Can you work these out from the drawing? Everything is in mm from the part's minimum corner. Give positions to 0.01 mm unless a question says otherwise; leave off trailing zeros. Write each loop counter-clockwise with the first axis right and the second up, starting at its lowest first coordinate (ties: lowest second). Pieces come first, ordered by that corner, then holes. Notation, with made-up numbers: (2, 66.25) - (59, 66.25) arc R24 ccw to (59, 95.25) - close; hole circle Ø11 at (-37, 67.25). An arc over 180 degrees is marked (long way). Use a Markdown table: item, result. Add a question column.
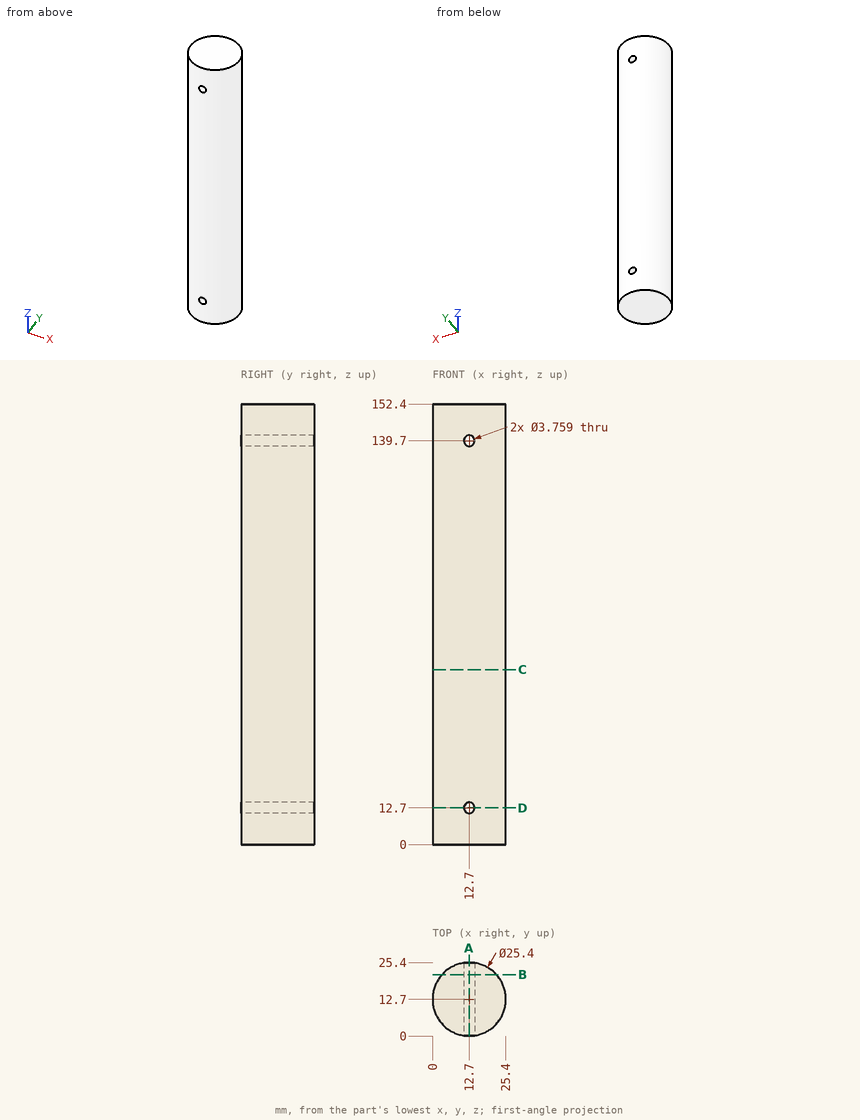
Q1. Suppose I cut it at C-C (z = 60.5). Please give me the cut outline in (x, y).
Q2. If I drill on probe 1 along Z at (x, y) = (12.7, 20); probe 2 along X at (y, z) = (12, 16); probe 3 along X at (y, z) = (17, 130), over which ranges is the centre line in solid material (lowest first)? Write a range as [from, to].
Q3. Suppose I cut it at A-A (x = 12.7). Please give me the cut outline in (y, z).
Q4. I'm going to push flat-ended pins straight in: P1, Ø5, axis at x = 2.5, z = 72.5, coming from the -Y side; P2, Ø2.5, axis at x = 12.7, z = 139.7, coming from the -Y side; P3, Ø6, axis at x = 3.5, z = 50.5, coming from the -Y side; P4, Ø10, axis at y = 5.5, z = 62.5, coming from the -X side. Where does each tip first touch, or does it pass through?
Q5. Suppose I cut it at D-D (z = 12.7). Please give me the cut outline in (x, y).
Q6. Suppose I cut it at B-B (y = 21.25). Please give me the cut outline in (x, z), and give its area (3 significant figures).
Derived:
| question | item | result |
|---|---|---|
| 1 | outline | circle Ø25.4 at (12.7, 12.7) |
| 2 | probe 1 | [0, 10.82], [14.58, 137.82], [141.58, 152.4] |
| 2 | probe 2 | [0.02, 25.38] |
| 2 | probe 3 | [0.75, 24.65] |
| 3 | outline | (0, 0) - (25.4, 0) - (25.4, 10.82) - (0, 10.82) - close; (0, 14.58) - (25.4, 14.58) - (25.4, 137.82) - (0, 137.82) - close; (0, 141.58) - (25.4, 141.58) - (25.4, 152.4) - (0, 152.4) - close |
| 4 | P1 | y = 2.6 |
| 4 | P2 | through |
| 4 | P3 | y = 1.62 |
| 4 | P4 | x = 0.19 |
| 5 | outline | (10.82, 0.14) - (10.82, 25.26) arc R12.7 ccw to start; (14.58, 0.14) arc R12.7 ccw to (14.58, 25.26) - close |
| 6 | outline | (3.31, 0) - (22.09, 0) - (22.09, 152.4) - (3.31, 152.4) - close; hole circle Ø3.76 at (12.7, 12.7); hole circle Ø3.76 at (12.7, 139.7) |
| 6 | area | 2,840 mm² |
